```python
from build123d import *

# Parameters (mm, degrees)
SKETCH1_W             = 140
SKETCH1_H             = 150
SKETCH1_R             = 2.75
SKETCH1_R_2           = 19.25
BOSS_EXTRUDE1_DEPTH   = 5
F_5_0MM_DOWEL_HOLE1_D = 5.5
F_6_0MM_DOWEL_HOLE2_D = 6.6


with BuildPart() as part:
    # Sketch1 → Boss-Extrude1 (new body)
    with BuildSketch(Plane.XY):
        with Locations((0, -11)):
            Rectangle(SKETCH1_W, SKETCH1_H)
        with Locations((23.5, 17.5)):
            Circle(SKETCH1_R, mode=Mode.SUBTRACT)
        with Locations((-23.5, 17.5)):
            Circle(SKETCH1_R, mode=Mode.SUBTRACT)
        with Locations((-23.5, -29.5)):
            Circle(SKETCH1_R, mode=Mode.SUBTRACT)
        with Locations((23.5, -29.5)):
            Circle(SKETCH1_R, mode=Mode.SUBTRACT)
        with Locations((0, -6)):
            Circle(SKETCH1_R_2, mode=Mode.SUBTRACT)
    extrude(amount=BOSS_EXTRUDE1_DEPTH)

    # Ø5.0mm Dowel Hole1 (through all)
    with Locations(Plane(origin=(60, -46, 0), x_dir=(-1, 0, 0), z_dir=(0, 0, -1))):
        with Locations((0, 0), (120, 0), (100, 0), (20, 0)):
            Hole(F_5_0MM_DOWEL_HOLE1_D / 2)

    # Ø6.0mm Dowel Hole2 (through all)
    with Locations(Plane(origin=(-50, 49, 5), x_dir=(1, 0, 0), z_dir=(0, 0, 1))):
        with Locations((0, 0), (100, 0), (100, -120), (0, -120)):
            Hole(F_6_0MM_DOWEL_HOLE2_D / 2)


solid = part.part
```
Work out the finished part from the listing and answer in its coordinate system (mm). Give positions to 0.01 mm unless a question says otherwise; leave off trailing zeros. Order: outer loops, then holes, each group sorted by start corner. A loop starts at its lowest first (then second) coordinate and runs counter-clockwise, first axis right, second up. Notation, with made-up numbers: (49, -36) - (77, -36) arc R8 ccw to (77, -25) - close; hole circle Ø9 at (48, 21.5). An arc over 180 degrees is marked (long way). One line per item, written item: value. Start each with the question number.
1. Section B-B, the plane z = 2.35 is taken. Count the separate pieces of the cut face and the enclosed holes in it, then the cut area to 3 significant figures.
2. For a pull along Y with two mould halves and no side action, classify faces 1 (the face through (-26.247, -29.379, 2.465)), 2 (the face through (-1, -86, 2)), 3 (the face through (70, -12, 2)), 4 (the face through (-62.027, -44.141, 2.535)) as released by +Y, released by -Y, zero draft, split by the parting line, or undercut.
3. Each of these flat-tipped pins is pushed along its axis until it touches: pin 1 Ø6.5 at (x, y) = (-60, -46) entering from -Z; pin 2 Ø23 at (x, y) = (0, -6) entering from -Z. Where does it stop, or does it pass through?
4. Consider line 1 (Y direction, x = -23.5, z = 1); line 2 (X direction, y = 47, z = 0.4); line 3 (X direction, y = -31, z = 3.3). Determine where each line is inside the solid, lowest interval first.
5. Section A-A, the plane y = -46 is taken. Write down the section's boundary in (x, z), then the cut area to 3 significant figures.
6. Section C-C, the plane x = 60 is taken. Write down the section's boundary in (y, z), then the cut area to 4 significant figures.
7. Section D-D, the plane y = 17.5 is taken. Write down the section's boundary in (x, z), then the cut area to 3 significant figures.
Filled sheet:
1. separate pieces: 1
1. enclosed holes: 13
1. area: 19,500 mm²
2. face 1: undercut
2. face 2: released by -Y
2. face 3: zero draft
2. face 4: undercut
3. pin 1: z = 0
3. pin 2: through
4. line 1: -86 to -32.25, -26.75 to 14.75, 20.25 to 64
4. line 2: -70 to -52.62, -47.38 to 47.38, 52.62 to 70
4. line 3: -70 to -25.8, -21.2 to 21.2, 25.8 to 70
5. outline: (-70, 0) - (-62.75, 0) - (-62.75, 5) - (-70, 5) - close; (-57.25, 0) - (-42.75, 0) - (-42.75, 5) - (-57.25, 5) - close; (-37.25, 0) - (37.25, 0) - (37.25, 5) - (-37.25, 5) - close; (42.75, 0) - (57.25, 0) - (57.25, 5) - (42.75, 5) - close; (62.75, 0) - (70, 0) - (70, 5) - (62.75, 5) - close
5. area: 590 mm²
6. outline: (-86, 0) - (-48.75, 0) - (-48.75, 5) - (-86, 5) - close; (-43.25, 0) - (64, 0) - (64, 5) - (-43.25, 5) - close
6. area: 722.5 mm²
7. outline: (-70, 0) - (-26.25, 0) - (-26.25, 5) - (-70, 5) - close; (-20.75, 0) - (20.75, 0) - (20.75, 5) - (-20.75, 5) - close; (26.25, 0) - (70, 0) - (70, 5) - (26.25, 5) - close
7. area: 645 mm²
